from build123d import *

# Parameters (mm, degrees)
SKETCH1_W           = 28
SKETCH1_H           = 6
BOSS_EXTRUDE1_DEPTH = 2
SKETCH2_W           = 7
SKETCH2_H           = 6
BOSS_EXTRUDE2_DEPTH = 16
SKETCH3_W           = 6
SKETCH3_H           = 2
BOSS_EXTRUDE3_DEPTH = 14
CUT_EXTRUDE1_DEPTH  = 24.579652245
SKETCH5_W           = 28
SKETCH5_H           = 6
BOSS_EXTRUDE4_DEPTH = 22
CUT_EXTRUDE2_DEPTH  = 30
CUT_EXTRUDE3_DEPTH  = 30
FILLET1_R           = 2


with BuildPart() as part:
    # Sketch1 → Boss-Extrude1 (new body)
    with BuildSketch(Plane(origin=(0, 0, 0), x_dir=(1, 0, 0), z_dir=(0, 1, 0))):
        Rectangle(SKETCH1_W, SKETCH1_H)
    extrude(amount=BOSS_EXTRUDE1_DEPTH)

    # Sketch2 → Boss-Extrude2 (add)
    with BuildSketch(Plane(origin=(0, 2, 0), x_dir=(1, 0, 0), z_dir=(0, 1, 0))):
        with Locations((-10.5, 0)):
            Rectangle(SKETCH2_W, SKETCH2_H)
        with Locations((10.5, 0)):
            Rectangle(SKETCH2_W, SKETCH2_H)
    extrude(amount=BOSS_EXTRUDE2_DEPTH)

    # Sketch3 → Boss-Extrude3 (add)
    with BuildSketch(Plane(origin=(-7, 0, 0), x_dir=(0, 0, -1), z_dir=(1, 0, 0))):
        with Locations((0, 17)):
            Rectangle(SKETCH3_W, SKETCH3_H)
    extrude(amount=BOSS_EXTRUDE3_DEPTH)

    # Sketch4 → Cut-Extrude1 (cut, through all)
    with BuildSketch(Plane(origin=(0, 0, -3), x_dir=(-1, 0, 0), z_dir=(0, 0, -1))):
        Polygon((-9, 18), (-14, 18), (-14, 2), align=None)
        Polygon((9, 18), (14, 18), (14, 2), align=None)
    extrude(amount=-CUT_EXTRUDE1_DEPTH, mode=Mode.SUBTRACT)

    # Sketch5 → Boss-Extrude4 (add)
    with BuildSketch(Plane.XZ):
        Rectangle(SKETCH5_W, SKETCH5_H)
    extrude(amount=BOSS_EXTRUDE4_DEPTH)

    # Sketch6 → Cut-Extrude2 (cut)
    with BuildSketch(Plane(origin=(14, 0, 0), x_dir=(0, 0, -1), z_dir=(1, 0, 0))):
        Polygon((3, 0), (-3, -22), (3, -22), align=None)
    extrude(amount=-CUT_EXTRUDE2_DEPTH, mode=Mode.SUBTRACT)

    # Sketch7 → Cut-Extrude3 (cut)
    with BuildSketch(Plane(origin=(14, 0, 0), x_dir=(0, 0, -1), z_dir=(1, 0, 0))):
        Polygon((-3, -22), (-3, -20), (-2.454545455, -20), align=None)
    extrude(amount=-CUT_EXTRUDE3_DEPTH, mode=Mode.SUBTRACT)

    # Fillet1
    fillet1_edges = [part.edges().sort_by_distance(p)[0] for p in [
        (0, 2, -3),
    ]]
    fillet(fillet1_edges, radius=FILLET1_R - 0.0001)  # a hair under: the kernel refuses the full size


solid = part.part
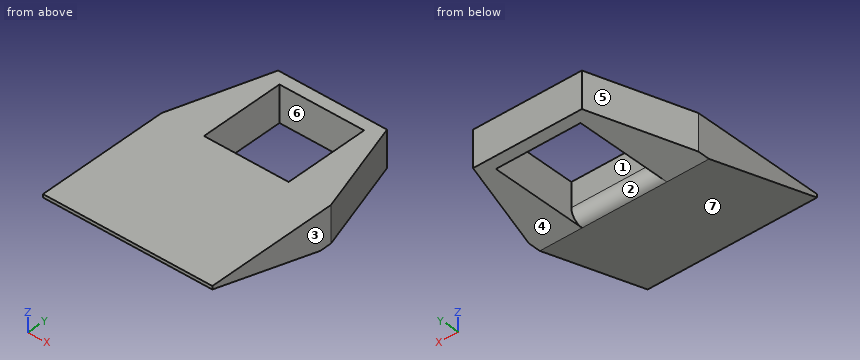
Verification items for the finished model (mm, model axes). Face numbers are marked on the shaded views. A direction names the side the tool comes from. Round coordinates to 2 decimals unless told otherwise and drop trailing zeros. Loops run counter-clockwise (first coordinate to the right, second up) from the corner with the lowest first, then second, coordinate; pieces in that order, holes last. Notation, with made-up numbers: (58, 26) - (104, 26) arc R10 cw to (104, 39) - close; hole circle Ø5 at (42.25, -31). An arc over 180 degrees is marked (long way). Use a Markdown table: item, result. Add a question column.
1. Section check A-A, the plane z = 0.3. Record the boundary of the cut face in (x, y), plus the area to 3 significant figures.
2. Thickness scan on probe 1 along Y at (x, z) = (-0.75, 2.6); probe 2 along X at (y, z) = (8.5, 1.7); probe 3 along X at (y, z) = (7, 1.25). Record the ranges inside material, lowest first. Write a range as [from, to].
3. Section check C-C, the plane y = 12. Record the boundary of the cut face in (x, z) (3 decimals).
4. Section check D-D, the plane z = 2.05. Record the boundary of the cut face in (x, y), plus the area to 3 significant figures.
5. Release check for a two-part mould opening along Y. For the marked faces 4, 5, 6 and 7 record: released by +Y, released by -Y, zero draft, split by the parting line, or undercut.
6. Access from +Z, -Z, +X, -X, +Y, -Y to the whole of each face (thin tool, end or side, straight path). Record for the marked faces 1, 2 and 3.
7. Gauge pin test, flat ends, axial feed: pin 1 (1.8 mm diameter, centred on y = 5, z = 1, fed in from -X); pin 2 (3 mm diameter, centred on y = 8, z = -0.5, fed in from -X); pin 3 (1.8 mm diameter, centred on y = 5, z = 1.5, fed in from +X). Record the tip position at first contact, or that the pin passes through.
Checks:
| question | item | result |
|---|---|---|
| 1 | outline | (-14, -12.1) - (14, -12.1) - (14, 2) - (9, 18) - (-9, 18) - (-14, 2) - close; hole (-7, 2) - (7, 2) - (7, 16) - (-7, 16) - close |
| 1 | area | 567 mm^2 |
| 2 | probe 1 | y = [-20, 2], [16, 18] |
| 2 | probe 2 | x = [-11.97, -7], [7, 11.97] |
| 2 | probe 3 | x = [-12.44, -7], [7, 12.44] |
| 3 | outline | (-10.875, -3) - (-7, -3) - (-7, 3) - (-10.875, 3) - close; (7, -3) - (10.875, -3) - (10.875, 3) - (7, 3) - close |
| 4 | outline | (-14, -18.52) - (14, -18.52) - (14, 2) - (9, 18) - (-9, 18) - (-14, 2) - close; hole (-7, 2) - (7, 2) - (7, 16) - (-7, 16) - close |
| 4 | area | 746 mm^2 |
| 5 | face 4 | zero draft |
| 5 | face 5 | released by +Y |
| 5 | face 6 | undercut |
| 5 | face 7 | released by -Y |
| 6 | face 1 | +Z, -Z |
| 6 | face 2 | -Z |
| 6 | face 3 | +Z, -Z, +X, +Y, -Y |
| 7 | pin 1 | stops at x = -13.34 |
| 7 | pin 2 | stops at x = -12.59 |
| 7 | pin 3 | stops at x = 13.34 |
